from build123d import *

# Parameters (mm, degrees)
F1_DEPTH = 100
F3_DEPTH = 105.41


with BuildPart() as f1:
    # F0 (on Top) → F1 (new body)
    with BuildSketch(Plane.XY):
        Polygon((35.355339, 35.355339), (0, 50), (-35.355339, 35.355339), (-50, 0), (-35.355339, -35.355339), (0, -50), (35.355339, -35.355339), (50, 0), align=None)
    extrude(amount=F1_DEPTH)

    # F2 (on Top) → F3 (cut)
    with BuildSketch(Plane.XY):
        Polygon((-40, 0), (-28.284271, -28.284271), (0, -40), (28.284271, -28.284271), (40, 0), (28.284271, 28.284271), (0, 40), (-28.284271, 28.284271), align=None)
    extrude(amount=F3_DEPTH, mode=Mode.SUBTRACT)


solid = f1.part
CAD build for the part. Positions are in the model's coordinates, mm. A direction names the side the tool comes from. Give positions to 0.01 mm unless a question says otherwise; leave off trailing zeros. Loops run counter-clockwise (first coordinate to the right, second up) from the corner with the lowest first, then second, coordinate; pieces in that order, holes last. Notation, with made-up numbers: M 35,75.5 L 68,75.5 A31 ccw 68,112.5 Z; hole C 47.5,-31.5 d3. An arc over 180 degrees is marked long. Answer in a Markdown table with one row per item. Add a question column.
Item 1: Probe probe 1 along Y at (x, z) = (0, 6.5); probe 2 along X at (y, z) = (12.5, 12); probe 3 along Y at (x, z) = (-8.5, 94.5). List the from-to ranges inside material, lowest first.
Item 2: Mould opens along Y. For faces 3 (the face through (-14.34, -34.06, 49.3)), 4 (the face through (17.43, -42.78, 49.3)), 5 (the face through (-34.224, -13.944, 49.3)), 6 (the face through (-17.43, 42.78, 49.3)) say: +Y half, -Y half, draft (parallel to the pull), parting line (faces both ways), or undercut.
Item 3: Tool access for faces 1 (the face through (42.575, -17.925, 49.3)), 2 (the face through (-13.944, 34.224, 49.3)): list every direction of +Z, -Z, +X, -X, +Y, -Y with a clear straight run to the whole face (end or side of a thin tool).
Item 4: Band-saw the part on B-B on x = 16. Give the cut face in (y, z), then the cut area to 3 significant figures.
Item 5: Band-saw the part on D-D on x = 44. Give the cut face in (y, z).
Item 6: Drop flat-ended pins along their axis: P1, Ø2, axis at x = 27.5, z = 29, coming from the -Y side; P2, Ø8, axis at y = -32.5, z = 70, coming from the -X side; P3, Ø2, axis at x = -32, z = 84, coming from the -Y side. Give the stop position or say it passes through.
Item 7: Band-saw the part on C-C on y = -17.5. Give the cut face in (x, z), then the cut area to 3 significant figures.
Item 8: Band-saw the part on A-A on z = 62.5. Give the cut face in (x, y), then the cut area to 3 significant figures.
Reply:
| question | item | result |
|---|---|---|
| 1 | probe 1 | y = -50 to -40, 40 to 50 |
| 1 | probe 2 | x = -44.82 to -34.82, 34.82 to 44.82 |
| 1 | probe 3 | y = -46.48 to -36.48, 36.48 to 46.48 |
| 2 | face 3 | undercut |
| 2 | face 4 | -Y half |
| 2 | face 5 | undercut |
| 2 | face 6 | +Y half |
| 3 | face 1 | +Z, -Z, +X, -Y |
| 3 | face 2 | +Z, -Z |
| 4 | outline | M -43.37,0 L -33.37,0 L -33.37,100 L -43.37,100 Z; M 33.37,0 L 43.37,0 L 43.37,100 L 33.37,100 Z |
| 4 | area | 2,000 mm^2 |
| 5 | outline | M -14.49,0 L 14.49,0 L 14.49,100 L -14.49,100 Z |
| 6 | P1 | stops at y = -39.02 |
| 6 | P2 | stops at x = -38.19 |
| 6 | P3 | stops at y = -37.16 |
| 7 | outline | M -42.75,0 L -32.75,0 L -32.75,100 L -42.75,100 Z; M 32.75,0 L 42.75,0 L 42.75,100 L 32.75,100 Z |
| 7 | area | 2,000 mm^2 |
| 8 | outline | M -50,0 L -35.36,-35.36 L 0,-50 L 35.36,-35.36 L 50,0 L 35.36,35.36 L 0,50 L -35.36,35.36 Z; hole M -40,0 L -28.28,-28.28 L 0,-40 L 28.28,-28.28 L 40,0 L 28.28,28.28 L 0,40 L -28.28,28.28 Z |
| 8 | area | 2,550 mm^2 |
